Model file for the job. Use its own axes, mm. A direction names the side the tool comes from. Coordinates: 2 decimals unless noted, no trailing zeros. Loops run counter-clockwise (first coordinate to the right, second up) from the corner with the lowest first, then second, coordinate; pieces in that order, holes last.
from build123d import *

# Parameters (mm, degrees)
ESQUISSE2_W             = 190
ESQUISSE2_H             = 30
BOSS_EXTRU_1_DEPTH      = 2
ESQUISSE3_W             = 128
ESQUISSE3_H             = 1.2
BOSS_EXTRU_2_DEPTH      = 38
CHANFREIN1_SIZE         = 10
CONG_1_R                = 2
ESQUISSE4_R             = 1.6
ENL_V_MAT_EXTRU_1_DEPTH = 41
CONG_2_R                = 10


with BuildPart() as part:
    # Esquisse2 → Boss.-Extru.1 (new body)
    with BuildSketch(Plane(origin=(0, 0, 0), x_dir=(1, 0, 0), z_dir=(0, 1, 0))):
        Rectangle(ESQUISSE2_W, ESQUISSE2_H)
    extrude(amount=BOSS_EXTRU_1_DEPTH)

    # Esquisse3 → Boss.-Extru.2 (add)
    with BuildSketch(Plane.XZ):
        with Locations((0, 14.4)):
            Rectangle(ESQUISSE3_W, ESQUISSE3_H)
    extrude(amount=BOSS_EXTRU_2_DEPTH)

    # Chanfrein1
    chanfrein1_edges = [part.edges().sort_by_distance(p)[0] for p in [
        (95, 1, 15),
        (-95, 1, 15),
    ]]
    chamfer(chanfrein1_edges, length=CHANFREIN1_SIZE)

    # Congé1
    cong_1_edges = [part.edges().sort_by_distance(p)[0] for p in [
        (95, 1, 5),
        (-85, 1, 15),
        (85, 1, 15),
        (-95, 1, 5),
    ]]
    fillet(cong_1_edges, radius=CONG_1_R)

    # Esquisse4 → Enlèv. mat.-Extru.1 (cut, through all)
    with BuildSketch(Plane(origin=(0, 2, 0), x_dir=(1, 0, 0), z_dir=(0, 1, 0))):
        with Locations((-80, -5)):
            Circle(ESQUISSE4_R)
        with Locations((80, -5)):
            Circle(ESQUISSE4_R)
    extrude(amount=-ENL_V_MAT_EXTRU_1_DEPTH, mode=Mode.SUBTRACT)

    # Congé2
    cong_2_edges = [part.edges().sort_by_distance(p)[0] for p in [
        (0, 0, 13.8),
    ]]
    fillet(cong_2_edges, radius=CONG_2_R)


solid = part.part
Q1. Flat gauge pins, fed straight in: P1, Ø2, axis at x = 41, z = 3, coming from the -Y side; P2, Ø1.9, axis at x = 80, z = 5, coming from the +Y side; P3, Ø10, axis at x = -10, z = 4, coming from the -Y side; P4, Ø15, axis at x = -44.5, z = 3.5, coming from the -Y side. Where does each tip first touch, or does it go through?
Answers:
P1: stops at y = 0
P2: passes through
P3: stops at y = -1.46
P4: stops at y = -3.06
Q2. Slice it at C-C (y = -7). List the corners of the cut face in (x, z).
Answers:
outline: (-64, 13.34) - (64, 13.34) - (64, 15) - (-64, 15) - close
Q3. Mould opens along X. For faces 1 (the cylindrical face through (-78.474, 1.014, 4.519)), 2 (the flat face through (-1, 2, 0)), 3 (the flat face through (64, -13, 14)) say: +X half, -X half, draft (parallel to the pull), parting line (faces both ways), or undercut.
Answers:
face 1: undercut
face 2: draft
face 3: +X half
Q4. Slice it at D-D (z = -9.25). List the corners of the cut face in (x, y).
Answers:
outline: (-95, 0) - (95, 0) - (95, 2) - (-95, 2) - close
Q5. Slice it at A-A (x = 80). List the corners of the cut face in (y, z).
Answers:
outline: (0, -15) - (2, -15) - (2, 3.4) - (0, 3.4) - close; (0, 6.6) - (2, 6.6) - (2, 15) - (0, 15) - close
Q6. Which spindle directions (+Z, -Z, +X, -X, +Y, -Y) get a long thin tool onto all of the face, cutting with end or side? Do faces 4 (the flat face through (-1, -18, 15)), 5 (the flat face through (-64, -13, 14)), 6 (the flat face through (-1, -24, 13.8)). Say none if no direction does.
Answers:
face 4: +Z, +X, -X, +Y, -Y
face 5: +Z, -Z, -X, -Y
face 6: -Z, +X, -X, -Y
Q7. Slice it at B-B (x = -57). List the corners of the cut face in (y, z), and give its area (3 significant figures).
Answers:
outline: (-38, 13.8) - (-10, 13.8) arc R10 cw to (0, 3.8) - (0, -15) - (2, -15) - (2, 15) - (-38, 15) - close
area: 127 mm2
Q8. Drill centre lines: line 1 (Z direction, x = -80, y = 1); line 2 (X direction, y = 0.85, z = 5); line 3 (Y direction, x = 20.5, z = 1.25). Where is each one in solid material? Low to high.
Answers:
line 1: z = -15 to 3.4, 6.6 to 15
line 2: x = -94.82 to -81.6, -78.4 to 78.4, 81.6 to 94.82
line 3: y = 0 to 2
